For this review, use the dimensioned drawing (mm, ordinates from the lowest corner) and the shaded views. Coordinates: 2 decimals unless noted, no trailing zeros. Loops run counter-clockwise (first coordinate to the right, second up) from the corner with the lowest first, then second, coordinate; pieces in that order, holes last. Notation, with made-up numbers: M -15,4.5 L 2,4.5 A15 ccw 2,10.5 Z; hole C 7,-23.75 d2. An arc over 180 degrees is marked long. One line per item, written item: value.
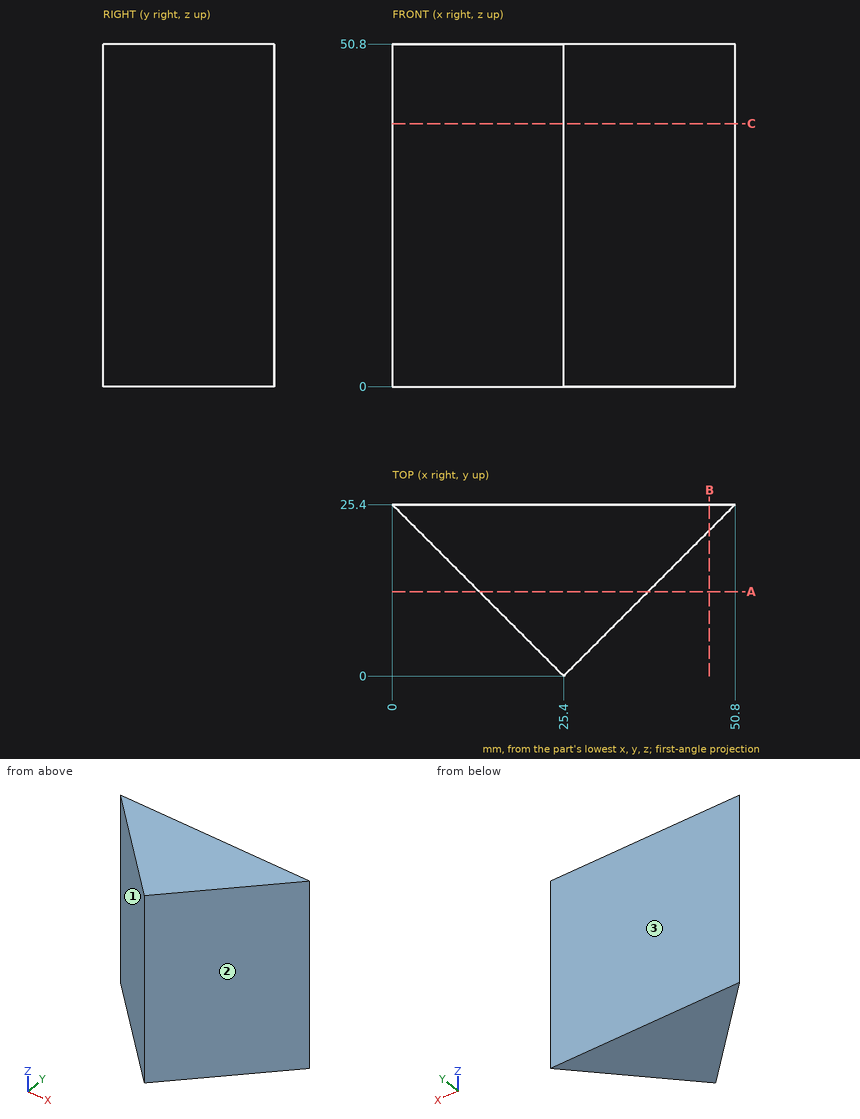
(1) We need section B-B on x = 47. State the section outline as (y, z) points.
Reply:
outline: M 21.6,0 L 25.4,0 L 25.4,50.8 L 21.6,50.8 Z
(2) Mouldability with a two-part tool opening along X and no side actions: class the marked faces 1, 2 and 3 as released by +X, released by -X, zero draft, split by the parting line, or undercut.
Reply:
face 1: released by -X
face 2: released by +X
face 3: zero draft
(3) Insertion check: pin 1 (8 mm diameter, centred on x = 43.5, y = 15.5, fed in from -Z); pin 2 (2 mm diameter, centred on y = 7, z = 32, fed in from +X); pin 3 (8 mm diameter, centred on y = 6.5, z = 27, fed in from -X); pin 4 (3 mm diameter, centred on x = 41.5, z = 27.5, fed in from -Y). Each pin has a flat end and moves straight along its axis. Give the tip position at first contact, or say it passes through.
Reply:
pin 1: stops at z = 0
pin 2: stops at x = 33.4
pin 3: stops at x = 14.9
pin 4: stops at y = 14.6
(4) To check wall thickness, follow line 1 along X through (y, z) = (8, 33.5); line 2 along Y through (x, z) = (27, 34); line 3 along X through (y, z) = (19, 42.5). State the ranges of each line that lie inside material, in increasing order. Write a range as [from, to].
Reply:
line 1: x = [17.4, 33.4]
line 2: y = [1.6, 25.4]
line 3: x = [6.4, 44.4]
(5) We need section C-C on z = 39. State the section outline as (x, y) points.
Reply:
outline: M 0,25.4 L 25.4,0 L 50.8,25.4 Z
(6) We need section A-A on y = 12.5. State the section outline as (x, z) points, then the cut area to 3 significant figures.
Reply:
outline: M 12.9,0 L 37.9,0 L 37.9,50.8 L 12.9,50.8 Z
area: 1,270 mm2
